For this review, take the finished solid that the model builds, in its own axes (mm). Face numbers are marked on the shaded views. A direction names the side the tool comes from. Round coordinates to 2 decimals unless told otherwise and drop trailing zeros. Order: outer loops, then holes, each group sorted by start corner. A loop starts at its lowest first (then second) coordinate and runs counter-clockwise, first axis right, second up. Notation, with made-up numbers: M 7,-4.5 L 31,-4.5 A24 cw 31,12.5 Z; hole C 20.25,41.25 d6. An arc over 180 degrees is marked long. Write item = value, one per line. Start each with the question number.
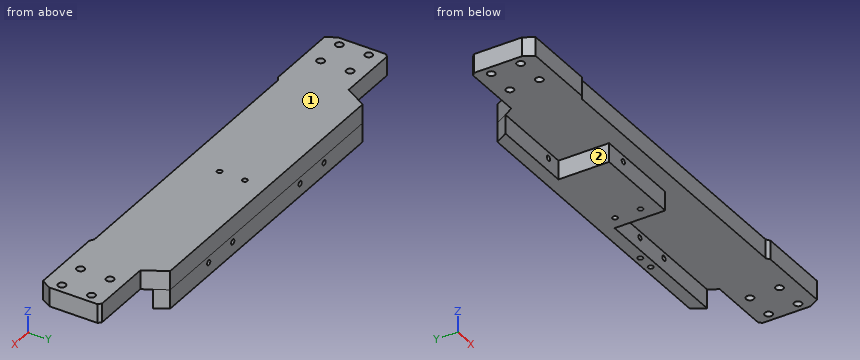
from build123d import *
from build123d.topology import SkipClean

# Parameters (mm, degrees)
SKETCH1_R               = 3
SKETCH1_R_2             = 2
BOSS_EXTRUDE1_DEPTH     = 15
BOSS_EXTRUDE2_START     = 15
SKETCH3_W               = 70
SKETCH3_H               = 40
SKETCH3_R               = 2
BOSS_EXTRUDE2_DEPTH     = 15
SKETCH4_R               = 2
CUT_EXTRUDE1_DEPTH      = 193.072300906
ESQUISSE1_R             = 2
ENL_V_MAT_EXTRU_1_DEPTH = 10


with BuildPart() as part:
    # Sketch1 → Boss-Extrude1 (new body)
    with BuildSketch(Plane.XY):
        Polygon((-114.627718677, 0), (114.627718677, 0), (117.5, -2), (175.5, -2), (180, 5.794228634), (180, 43.794228634), (177.794228634, 46), (130, 46), (120, 63.320508076), (-120, 63.320508076), (-130, 46), (-177.794228634, 46), (-180, 43.794228634), (-180, 5.794228634), (-175.5, -2), (-117.5, -2), align=None)
        with Locations((-173, 34.625)):
            Circle(SKETCH1_R, mode=Mode.SUBTRACT)
        with Locations((-149.75, 34.625)):
            Circle(SKETCH1_R, mode=Mode.SUBTRACT)
        with Locations((-173, 11.375)):
            Circle(SKETCH1_R, mode=Mode.SUBTRACT)
        with Locations((-149.75, 11.375)):
            Circle(SKETCH1_R, mode=Mode.SUBTRACT)
        with Locations((149.75, 34.625)):
            Circle(SKETCH1_R, mode=Mode.SUBTRACT)
        with Locations((173, 34.625)):
            Circle(SKETCH1_R, mode=Mode.SUBTRACT)
        with Locations((149.75, 11.375)):
            Circle(SKETCH1_R, mode=Mode.SUBTRACT)
        with Locations((173, 11.375)):
            Circle(SKETCH1_R, mode=Mode.SUBTRACT)
        with Locations((0, 46.320508076)):
            Circle(SKETCH1_R_2, mode=Mode.SUBTRACT)
        with Locations((0, 26.320508076)):
            Circle(SKETCH1_R_2, mode=Mode.SUBTRACT)
    extrude(amount=BOSS_EXTRUDE1_DEPTH)

    # Sketch3 → Boss-Extrude2 (add)
    # profile 1 of 2: a face of its own
    with SkipClean():  # the faces are left unmerged after this step: merging them gives an invalid solid
        with BuildSketch(Plane(origin=(0, 0, 0), x_dir=(-1, 0, 0), z_dir=(0, 0, -1)).offset(BOSS_EXTRUDE2_START)):
            with Locations((24.627718677, 33.320508076)):
                Rectangle(SKETCH3_W, SKETCH3_H)
            with Locations((0, 26.320508076)):
                Circle(SKETCH3_R, mode=Mode.SUBTRACT)
            with Locations((0, 46.320508076)):
                Circle(SKETCH3_R, mode=Mode.SUBTRACT)
        # profile 2 of 2: a face of its own
        with BuildSketch(Plane(origin=(0, 0, 0), x_dir=(-1, 0, 0), z_dir=(0, 0, -1)).offset(BOSS_EXTRUDE2_START)):
            Polygon((120, 63.320508076), (-120, 63.320508076), (-125.773502692, 53.320508076), (-10.372281323, 53.320508076), (59.627718677, 53.320508076), (125.773502692, 53.320508076), align=None)
        extrude(amount=-BOSS_EXTRUDE2_DEPTH)

    # Sketch4 → Cut-Extrude1 (cut, through all)
    with SkipClean():  # the faces are left unmerged after this step: merging them gives an invalid solid
        with BuildSketch(Plane(origin=(0, 63.320508076, 0), x_dir=(1, 0, 0), z_dir=(0, 1, 0))):
            with Locations(Location((-72, 5, 0), (0, 0, 180))):
                Circle(SKETCH4_R)
            with Locations(Location((-42, 5, 0), (0, 0, 180))):
                Circle(SKETCH4_R)
            with Locations((42, 5)):
                Circle(SKETCH4_R)
            with Locations((72, 5)):
                Circle(SKETCH4_R)
        extrude(amount=-CUT_EXTRUDE1_DEPTH, mode=Mode.SUBTRACT)

    # Esquisse1 → Enlèv. mat.-Extru.1 (cut)
    with SkipClean():  # the faces are left unmerged after this step: merging them gives an invalid solid
        with BuildSketch(Plane(origin=(0, 0, -15), x_dir=(-1, 0, 0), z_dir=(0, 0, -1))):
            with Locations((-50.372281323, 58.320508076)):
                Circle(ESQUISSE1_R)
            with Locations((-63.372281323, 58.320508076)):
                Circle(ESQUISSE1_R)
        extrude(amount=-ENL_V_MAT_EXTRU_1_DEPTH, mode=Mode.SUBTRACT)


solid = part.part
(1) For line 1 along Y through (x, z) = (-149.75, 4) (3 decimals); line 2 along Y through (x, z) = (0, 3.5); line 3 along X through (y, z) = (13.5, -5.25), list the stretches that pass through material, from the lowest coordinate up.
(2) We need section D-D, the plane x = 30. Write out the cut boundary in (y, z), then the cut area to 3 significant figures.
(3) We need section C-C, the plane x = -36.5. Write out the cut boundary in (y, z).
(4) We need section A-A, the plane x = 149.75. Write out the cut boundary in (y, z) (3 decimals).
(5) For the marked faces 1 and 2, list the 3-axis set-ups (+Z, -Z, +X, -X, +Y, -Y) from which the entire face can be reached by the end or side of a thin tool; tool diameter is ignored.
(6) Insertion check: pin 1 (12 mm diameter, centred on y = 37.5, z = -7, fed in from +X); pin 2 (5 mm diameter, centred on y = 50.5, z = -11, fed in from -X); pin 3 (4.5 mm diameter, centred on x = 77.5, z = -7.5, fed in from -Y). Each pin has a flat end and moves straight along its axis. Give the tip position at first contact, or say it passes through.
(7) We need section B-B, the plane z = 4.5. State how many separate pieces and enclosed holes the cut face has, then the cut area to 3 significant figures.
Values:
q1.line_1 = -2 to 8.375, 14.375 to 31.625, 37.625 to 46
q1.line_2 = 0 to 24.32, 28.32 to 44.32, 48.32 to 63.32
q1.line_3 = -59.63 to -43.98, -40.02 to 10.37
q2.outline = M 0,0 L 53.32,0 L 53.32,-15 L 63.32,-15 L 63.32,15 L 0,15 Z
q2.area = 1,100 mm²
q3.outline = M 0,0 L 13.32,0 L 13.32,-15 L 63.32,-15 L 63.32,15 L 0,15 Z
q4.outline = M -2,0 L 8.375,0 L 8.375,15 L -2,15 Z; M 14.375,0 L 31.625,0 L 31.625,15 L 14.375,15 Z; M 37.625,0 L 46,0 L 46,15 L 37.625,15 Z
q5.face_1 = +Z, +X, -X, +Y, -Y
q5.face_2 = -Z, -X, -Y
q6.pin_1 = 10.37
q6.pin_2 = -59.63
q6.pin_3 = 53.32
q7.separate_pieces = 1
q7.enclosed_holes = 10
q7.area = 20,900 mm²
